Design review of the part built by this model. Coordinates are the model's own, in mm. Face numbers are marked on the shaded views. A direction names the side the tool comes from. Round coordinates to 2 decimals unless told otherwise and drop trailing zeros. Write each loop counter-clockwise with the first axis right and the second up, starting at its lowest first coordinate (ties: lowest second). Pieces come first, ordered by that corner, then holes. Notation, with made-up numbers: M 53.5,65 L 94.5,65 A26 ccw 94.5,95 Z; hole C 10.25,56 d9. An arc over 180 degrees is marked long. One line per question, with ' | ' between items. Start each with the question number.
Item 1: Insertion check: pin 1 Ø3 at (x, y) = (18.5, 1) entering from -Z; pin 2 Ø6 at (x, y) = (38, 8.5) entering from +Z; pin 3 Ø8 at (x, y) = (44.5, 0.5) entering from +Z. Each pin has a flat end and moves straight along its axis. Give the tip position at first contact, or say it passes through.
Item 2: For L1, parallel to Y at x = 41.5, z = 6; L2, parallel to Y at x = 8, z = 17; L3, parallel to Y at x = 36, z = 6.5, list the stretches that pass through material, from the lowest coordinate up.
Item 3: Add section D-D, the plane z = 10.25. Give the number of separate pieces and of enclosed holes in the cut face, and give its area (3 significant figures).
Item 4: Add section B-B, the plane z = 4.5. State the section outline as (x, y) points, and give its area (3 significant figures).
Item 5: Machinability: for the marked faces 1, 2 and 3, which of the approach directions +Z, -Z, +X, -X, +Y, -Y give a long, thin tool a straight path to every point of the face, cutting with its end or side? Answer none if there is none.
Item 6: Add section C-C, the plane x = 38. State the section outline as (y, z) points, and give its area (3 significant figures).
Item 7: Add section A-A, the plane y = 8.5. State the section outline as (x, z) points.
Item 8: Draft analysis for pull direction Y (two halves, no side actions). For the marked faces 4, 5 and 6, state which applies: released by +Y, released by -Y, zero draft, split by the parting line, or undercut.
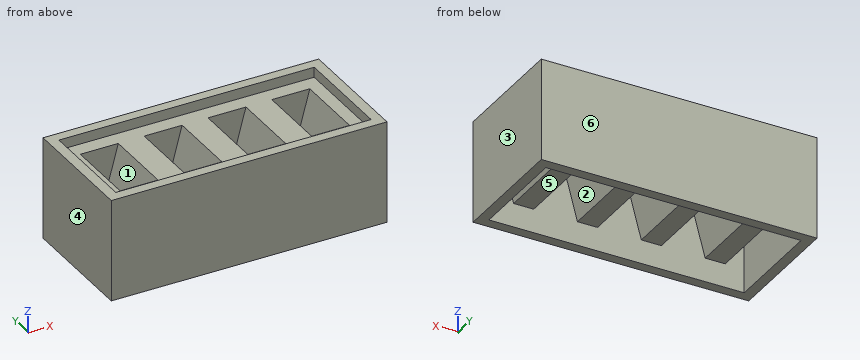
```python
from build123d import *

# Parameters (mm, degrees)
F1_DEPTH = 50
F3_DEPTH = 9
F4_DEPTH = 9
F5_W     = 20
F5_H     = 2
F5_H_2   = 16
F6_DEPTH = 2
F8_DEPTH = 2


# Not quite as in the source:
# - a feature names something its author has since deleted; it is built from what else it names


with BuildPart() as f1:
    # F0 (on Right) → F1 (new body)
    with BuildSketch(Plane.YZ):
        Polygon((10, 18), (7, 18), (7, 6), (0, 6), (-7, 6), (-7, 18), (-10, 18), (-10, 20), (-12, 20), (-12, 0), (-10, 0), (-10, 16), (-9, 16), (-9, 4), (0, 4), (9, 4), (9, 16), (10, 16), (10, 0), (12, 0), (12, 20), (10, 20), align=None)
    extrude(amount=F1_DEPTH)

    # F2 (on Front) → F3 (join, symmetric)
    with BuildSketch(Plane.XZ):
        Polygon((37.4974226119, 16), (38.5692193817, 16), (41.7846096908, 4), (45.7128129211, 4), (48.9282032303, 16), (50, 16), (50, 18), (49.4641016151, 18), (47.4641016151, 18), (44.248711306, 6), (43.248711306, 6), (40.0333209968, 18), (38.0333209968, 18), (37.4974226119, 18), (36.9615242271, 18), (34.9615242271, 18), (31.7461339179, 6), (30.7461339179, 6), (27.5307436087, 18), (25.5307436087, 18), (24.9948452239, 18), (24.458946839, 18), (22.458946839, 18), (19.2435565298, 6), (18.2435565298, 6), (15.0281662206, 18), (13.0281662206, 18), (12.4922678358, 18), (11.9563694509, 18), (9.9563694509, 18), (6.7409791417, 6), (5.7409791417, 6), (2.5255888326, 18), (0.5255888326, 18), (-0.0103095523, 18), (-0.0103095523, 16), (1.0614872174, 16), (4.2768775266, 4), (8.2050807569, 4), (11.4204710661, 16), (12.4922678358, 16), (13.5640646055, 16), (16.7794549147, 4), (20.707658145, 4), (23.9230484541, 16), (24.9948452239, 16), (26.0666419936, 16), (29.2820323028, 4), (33.210235533, 4), (36.4256258422, 16), align=None)
    extrude(amount=F3_DEPTH, both=True)

    # F2 (on Front) → F4 (cut, symmetric)
    with BuildSketch(Plane.XZ):
        Polygon((48.9282032303, 16), (45.7128129211, 4), (50, 4), (50, 16), align=None)
        Polygon((41.7846096908, 4), (38.5692193817, 16), (37.4974226119, 16), (36.4256258422, 16), (33.210235533, 4), (37.4974226119, 4), align=None)
        Polygon((24.9948452239, 4), (29.2820323028, 4), (26.0666419936, 16), (24.9948452239, 16), (23.9230484541, 16), (20.707658145, 4), align=None)
        Polygon((12.4922678358, 4), (16.7794549147, 4), (13.5640646055, 16), (12.4922678358, 16), (11.4204710661, 16), (8.2050807569, 4), align=None)
        Polygon((-0.0103095523, 4), (4.2768775266, 4), (1.0614872174, 16), (-0.0103095523, 16), align=None)
    extrude(amount=F4_DEPTH, both=True, mode=Mode.SUBTRACT)

    # F5 (on face) → F6 (join)
    with BuildSketch(Plane.YZ.offset(50)):
        with Locations((0, 19)):
            Rectangle(F5_W, F5_H)
        Polygon((-10, 20), (-12, 20), (-12, 0), (-10, 0), (-10, 16), (10, 16), (10, 0), (12, 0), (12, 20), (10, 20), (10, 18), (-10, 18), align=None)
        with Locations((0, 8)):
            Rectangle(F5_W, F5_H_2)
    extrude(amount=F6_DEPTH)

    # F7 (on face) → F8 (join)
    with BuildSketch(Plane(origin=(0, 0, 0), x_dir=(0, -1, 0), z_dir=(-1, 0, 0))):
        Polygon((12, 20), (10, 20), (10, 18), (9, 18), (9, 16), (10, 16), (10, 0), (12, 0), align=None)
        Polygon((10, 20), (-12, 20), (-12, 0), (10, 0), (10, 16), (9, 16), (9, 18), (10, 18), align=None)
    extrude(amount=F8_DEPTH)


solid = f1.part
```
Computed values:
1) pin 1: stops at z = 4 | pin 2: stops at z = 20 | pin 3: stops at z = 18
2) L1: y = -12 to -10, -9 to 9, 10 to 12 | L2: y = -12 to -7, 7 to 12 | L3: y = -12 to -10, 10 to 12
3) separate pieces: 5 | enclosed holes: 5 | area: 636 mm^2
4) outline: M -2,-12 L 52,-12 L 52,12 L -2,12 Z; M 4.14,-9 L 8.34,-9 L 8.34,9 L 4.14,9 Z; M 16.65,-9 L 20.84,-9 L 20.84,9 L 16.65,9 Z; M 29.15,-9 L 33.34,-9 L 33.34,9 L 29.15,9 Z; M 41.65,-9 L 45.85,-9 L 45.85,9 L 41.65,9 Z; hole M 0,-10 L 50,-10 L 50,10 L 0,10 Z | area: 598 mm^2
5) face 1: +Z | face 2: -Z | face 3: +Z, -Z, +X, +Y, -Y
6) outline: M -12,0 L -10,0 L -10,16 L 10,16 L 10,0 L 12,0 L 12,20 L 10,20 L 10,18 L -10,18 L -10,20 L -12,20 Z | area: 120 mm^2
7) outline: M -2,0 L 0,0 L 0,16 L 1.06,16 L 4.28,4 L 8.21,4 L 11.42,16 L 13.56,16 L 16.78,4 L 20.71,4 L 23.92,16 L 26.07,16 L 29.28,4 L 33.21,4 L 36.43,16 L 38.57,16 L 41.78,4 L 45.71,4 L 48.93,16 L 50,16 L 50,0 L 52,0 L 52,20 L 50,20 L 50,18 L 0,18 L 0,20 L -2,20 Z
8) face 4: zero draft | face 5: undercut | face 6: released by +Y
